from build123d import *

# Parameters (mm, degrees)
BOSS_EXTRUDE1_DEPTH = 3.175
CUT_EXTRUDE7_DEPTH  = 127


with BuildPart() as part:
    # Sketch1 → Boss-Extrude1 (new body)
    with BuildSketch(Plane.XY):
        Polygon((0, 266.7), (25.4, 292.1), (279.4, 292.1), (304.8, 266.7), (304.8, 0), (279.4, -25.4), (25.4, -25.4), (0, 0), align=None)
    extrude(amount=BOSS_EXTRUDE1_DEPTH)

    # Sketch4 → Cut-Extrude7 (cut)
    with BuildSketch(Plane.XY.offset(3.175)):
        with BuildLine():
            Line((50.258895016, 241.3), (120.933418015, 241.3))
            ThreePointArc((120.933418015, 241.3), (132.607750972, 236.464332957), (137.443418015, 224.79))
            Line((137.443418015, 224.79), (137.443418015, 177.875697945))
            ThreePointArc((137.443418015, 177.875697945), (132.607750972, 166.201364987), (120.933418015, 161.365697945))
            Line((120.933418015, 161.365697945), (50.258895016, 161.365697945))
            ThreePointArc((50.258895016, 161.365697945), (38.584562059, 166.201364987), (33.748895016, 177.875697945))
            Line((33.748895016, 177.875697945), (33.748895016, 224.79))
            ThreePointArc((33.748895016, 224.79), (38.584562059, 236.464332957), (50.258895016, 241.3))
        make_face()
        with BuildLine():
            Line((195.366803118, 241.3), (256.035491463, 241.3))
            ThreePointArc((256.035491463, 241.3), (266.070381863, 237.143412299), (270.226969564, 227.108521899))
            Line((270.226969564, 227.108521899), (270.226969564, 176.308521899))
            ThreePointArc((270.226969564, 176.308521899), (266.070381863, 166.273631498), (256.035491463, 162.117043797))
            Line((256.035491463, 162.117043797), (195.366803118, 162.117043797))
            ThreePointArc((195.366803118, 162.117043797), (185.331912718, 166.273631498), (181.175325017, 176.308521899))
            Line((181.175325017, 176.308521899), (181.175325017, 227.108521899))
            ThreePointArc((181.175325017, 227.108521899), (185.331912718, 237.143412299), (195.366803118, 241.3))
        make_face()
        with BuildLine():
            Line((121.145780521, 123.265697945), (46.236873468, 123.265697945))
            ThreePointArc((46.236873468, 123.265697945), (36.46177638, 119.216720157), (32.412798593, 109.44162307))
            Line((32.412798593, 109.44162307), (32.412798593, 39.224074875))
            ThreePointArc((32.412798593, 39.224074875), (36.46177638, 29.448977787), (46.236873468, 25.4))
            Line((46.236873468, 25.4), (121.551145478, 25.4))
            ThreePointArc((121.551145478, 25.4), (131.326242565, 29.448977787), (135.375220353, 39.224074875))
            Line((135.375220353, 39.224074875), (135.375220353, 109.44162307))
            ThreePointArc((135.375220353, 109.44162307), (131.183991006, 119.362876931), (121.145780521, 123.265697945))
        make_face()
        with BuildLine():
            Line((196.644821232, 124.017043797), (258.815551629, 124.017043797))
            ThreePointArc((258.815551629, 124.017043797), (269.182807745, 119.722785709), (273.477065833, 109.355529593))
            Line((273.477065833, 109.355529593), (273.477065833, 40.061514204))
            ThreePointArc((273.477065833, 40.061514204), (269.182807745, 29.694258088), (258.815551629, 25.4))
            Line((258.815551629, 25.4), (196.644821232, 25.4))
            ThreePointArc((196.644821232, 25.4), (186.277565116, 29.694258088), (181.983307028, 40.061514204))
            Line((181.983307028, 40.061514204), (181.983307028, 109.355529593))
            ThreePointArc((181.983307028, 109.355529593), (186.277565116, 119.722785709), (196.644821232, 124.017043797))
        make_face()
    extrude(amount=-CUT_EXTRUDE7_DEPTH, mode=Mode.SUBTRACT)


solid = part.part
CAD build for the part. Positions are in the model's coordinates, mm. A direction names the side the tool comes from. Coordinates: 2 decimals unless noted, no trailing zeros. Write each loop counter-clockwise with the first axis right and the second up, starting at its lowest first coordinate (ties: lowest second). Pieces come first, ordered by that corner, then holes. Notation, with made-up numbers: (2.25, 6.5) - (39.25, 6.5) arc R19 cw to (39.25, 40.5) - close; hole circle Ø8 at (82, 67.25). An arc over 180 degrees is marked (long way). Use a Markdown table: item, result. Add a question column.
Item 1: Band-saw the part on C-C, the plane x = 19. Give the cut face in (y, z) (3 decimals).
Item 2: Band-saw the part on D-D, the plane z = 2.45. Give the number of separate pieces and of enclosed holes in the cut face, and give its area (3 significant figures).
Item 3: 3-axis set-ups, long thin cutter, end or side, ignore diameter. For faces 4 (the face through (132.48, 236.59, 1.61)), 5 (the face through (155, 136, 3.175)): which of +Z, -Z, +X, -X, +Y, -Y reach the whole face in a straight line?
Item 4: Band-saw the part on B-B, the plane x = 97.5. Give the cut face in (y, z) (3 decimals).
Item 5: Band-saw the part on A-A, the plane y = 85. Give the cut face in (x, z) (3 decimals).
Item 6: Drill centre lines: L1, parallel to Y at x = 247.5, z = 0.6; L2, parallel to X at y = 48, z = 1.9; L3, parallel to Y at x = 87, z = 1.4. Where is each one in solid material? Low to high. Write a range as from..to.
Item 7: Mould opens along X. For faces 1 (the face through (155, 136, 0)), 2 (the face through (36.35, 29.56, 1.61)), 3 (the face through (12.5, 279.2, 1.6)) say: pulls with the +X half, pulls with the -X half, needs draft (parallel to the pull), parting line crosses it, or undercut.
Numbers:
| question | item | result |
|---|---|---|
| 1 | outline | (-19, 0) - (285.7, 0) - (285.7, 3.175) - (-19, 3.175) - close |
| 2 | separate pieces | 1 |
| 2 | enclosed holes | 4 |
| 2 | area | 61,800 mm2 |
| 3 | face 4 | +Z, -Z |
| 3 | face 5 | +Z, +X, -X, +Y, -Y |
| 4 | outline | (-25.4, 0) - (25.4, 0) - (25.4, 3.175) - (-25.4, 3.175) - close; (123.266, 0) - (161.366, 0) - (161.366, 3.175) - (123.266, 3.175) - close; (241.3, 0) - (292.1, 0) - (292.1, 3.175) - (241.3, 3.175) - close |
| 5 | outline | (0, 0) - (32.413, 0) - (32.413, 3.175) - (0, 3.175) - close; (135.375, 0) - (181.983, 0) - (181.983, 3.175) - (135.375, 3.175) - close; (273.477, 0) - (304.8, 0) - (304.8, 3.175) - (273.477, 3.175) - close |
| 6 | L1 | -25.4..25.4, 124.02..162.12, 241.3..292.1 |
| 6 | L2 | 0..32.41, 135.38..181.98, 273.48..304.8 |
| 6 | L3 | -25.4..25.4, 123.27..161.37, 241.3..292.1 |
| 7 | face 1 | needs draft |
| 7 | face 2 | undercut |
| 7 | face 3 | pulls with the -X half |
